Verification items for the finished model (mm, model axes). Face numbers are marked on the shaded views. A direction names the side the tool comes from. Give positions to 0.01 mm unless a question says otherwise; leave off trailing zeros. Write each loop counter-clockwise with the first axis right and the second up, starting at its lowest first coordinate (ties: lowest second). Pieces come first, ordered by that corner, then holes. Notation, with made-up numbers: (55.25, -3) -> (94.25, -3) arc R8 ccw to (94.25, 4) -> close; hole circle Ø1 at (46, 45). An arc over 180 degrees is marked (long way). Answer as CSV lines item,"result".
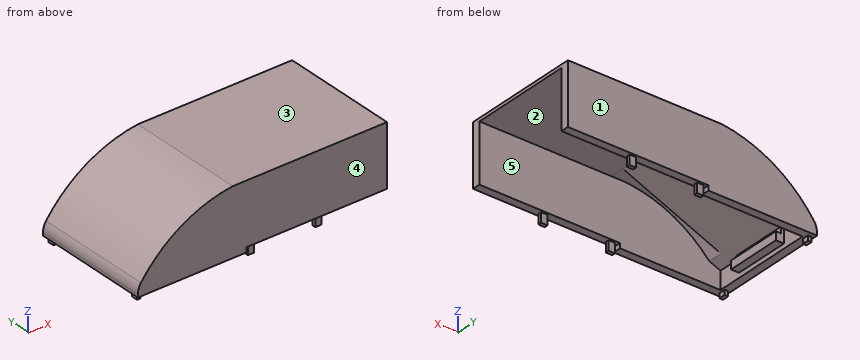
```python
from build123d import *

# Parameters (mm, degrees)
CROQUIS1_W              = 118
CROQUIS1_H              = 74
SALIENTE_EXTRUIR1_DEPTH = 36
CROQUIS2_W              = 36
CROQUIS2_H              = 64
CORTAR_EXTRUIR1_DEPTH   = 120
CORTAR_EXTRUIR3_DEPTH   = 102.257098517
SALIENTE_EXTRUIR2_DEPTH = 64
CORTAR_EXTRUIR4_DEPTH   = 9
CORTAR_EXTRUIR5_DEPTH   = 9
SALIENTE_EXTRUIR4_DEPTH = 5
CROQUIS14_W             = 50.5
CROQUIS14_H             = 3
CORTAR_EXTRUIR7_DEPTH   = 74
CROQUIS15_W             = 4
CROQUIS15_H             = 2.2
CROQUIS15_W_2           = 2.2
CROQUIS15_H_2           = 4
SALIENTE_EXTRUIR3_DEPTH = 6
REDONDEO1_R             = 10
SALIENTE_EXTRUIR5_DEPTH = 37
CROQUIS21_W             = 8
CROQUIS21_H             = 35
SALIENTE_EXTRUIR6_DEPTH = 5
CROQUIS22_W             = 2.9
CROQUIS22_H             = 35
CORTAR_EXTRUIR8_DEPTH   = 5
CROQUIS23_W             = 3.8
CROQUIS23_H             = 35
SALIENTE_EXTRUIR7_DEPTH = 1.9


with BuildPart() as part:
    # Croquis1 → Saliente-Extruir1 (new body)
    with BuildSketch(Plane.XY):
        Rectangle(CROQUIS1_W, CROQUIS1_H)
    extrude(amount=SALIENTE_EXTRUIR1_DEPTH)

    # Croquis2 → Cortar-Extruir1 (cut)
    with BuildSketch(Plane(origin=(59, 0, 0), x_dir=(0, 0, -1), z_dir=(1, 0, 0))):
        with Locations((-18, 0)):
            Rectangle(CROQUIS2_W, CROQUIS2_H)
    extrude(amount=-CORTAR_EXTRUIR1_DEPTH, mode=Mode.SUBTRACT)


with BuildPart() as cortar_extruir1_piece_1:
    # of the separate pieces the step leaves, piece 1, a body of its own (cortar_extruir1_pieces)
    add(part.part.solids().sort_by_distance((-59, 37, 0))[0])


with BuildPart() as cortar_extruir1_piece_2:
    # of the separate pieces the step leaves, piece 2, a body of its own (cortar_extruir1_pieces)
    add(part.part.solids().sort_by_distance((-59, -37, 0))[0])


with BuildPart() as cortar_extruir3_tool:
    # Croquis6 → Cortar-Extruir3 (new, through all)
    with BuildSketch(Plane.XZ.offset(37)):
        with BuildLine():
            Line((-59, 0), (-59, 36))
            Line((-59, 36), (0, 36))
            ThreePointArc((0, 36), (-33.535731191, 24.614115008), (-59, 0))
        make_face()
    extrude(amount=-CORTAR_EXTRUIR3_DEPTH)


with BuildPart() as cortar_extruir1_piece_1_1:
    add(cortar_extruir1_piece_1.part)

    # Cortar-Extruir3: cut by cortar_extruir3_tool
    add(cortar_extruir3_tool.part, mode=Mode.SUBTRACT)



with BuildPart() as cortar_extruir1_piece_2_1:
    add(cortar_extruir1_piece_2.part)

    # Cortar-Extruir3: cut by cortar_extruir3_tool
    add(cortar_extruir3_tool.part, mode=Mode.SUBTRACT)


with BuildPart() as cortar_extruir1_piece_1_2:
    add(cortar_extruir1_piece_1_1.part)

    add(cortar_extruir1_piece_2_1.part)  # Saliente-Extruir2 merges Cortar-Extruir1 piece 2
    # Croquis7 → Saliente-Extruir2 (add)
    with BuildSketch(Plane.XZ.offset(-32)):
        with BuildLine():
            Line((0, 36), (59, 36))
            Line((59, 36), (59, 34))
            Line((59, 34), (14, 34))
            Line((14, 34), (-54, 6))
            Line((-54, 6), (-54, 0))
            Line((-54, 0), (-59, 0))
            ThreePointArc((-59, 0), (-33.535731191, 24.614115008), (0, 36))
        make_face()
    extrude(amount=SALIENTE_EXTRUIR2_DEPTH)

    # Croquis8 → Cortar-Extruir4 (cut)
    with BuildSketch(Plane.XZ.offset(-32)):
        with BuildLine():
            Line((14, 34), (-46.937159353, 8.908228502))
            ThreePointArc((-46.937159353, 8.908228502), (-19.288572578, 28.30266844), (14, 34))
        make_face()
    extrude(amount=CORTAR_EXTRUIR4_DEPTH, mode=Mode.SUBTRACT)

    # Croquis13 → Cortar-Extruir5 (cut)
    with BuildSketch(Plane(origin=(0, -32, 0), x_dir=(1, 0, 0), z_dir=(0, 1, 0))):
        with BuildLine():
            Line((14, -34), (-46.936286689, -8.908587834))
            ThreePointArc((-46.936286689, -8.908587834), (-19.28805118, -28.302641518), (14, -34))
        make_face()
    extrude(amount=CORTAR_EXTRUIR5_DEPTH, mode=Mode.SUBTRACT)

    # Croquis17 → Saliente-Extruir4 (add)
    with BuildSketch(Plane(origin=(0, 0, 0), x_dir=(-1, 0, 0), z_dir=(0, 0, -1))):
        Polygon((-59, 37), (-59, 32), (54, 32), (54, -32), (-59, -32), (-59, -37), (59, -37), (59, 37), align=None)
    extrude(amount=SALIENTE_EXTRUIR4_DEPTH)

    # Croquis14 → Cortar-Extruir7 (cut)
    with BuildSketch(Plane.XZ.offset(37)):
        with Locations((33.75, -3.5)):
            Rectangle(CROQUIS14_W, CROQUIS14_H)
    extrude(amount=-CORTAR_EXTRUIR7_DEPTH, mode=Mode.SUBTRACT)

    # Croquis15 → Saliente-Extruir3 (add)
    with BuildSketch(Plane(origin=(0, 0, -2), x_dir=(-1, 0, 0), z_dir=(0, 0, -1))):
        with Locations((-54.5, 34.5)):
            Rectangle(CROQUIS15_W, CROQUIS15_H)
        with Locations((-54.5, -34.5)):
            Rectangle(CROQUIS15_W, CROQUIS15_H)
        with Locations((-12.5, 34.5)):
            Rectangle(CROQUIS15_W, CROQUIS15_H)
        with Locations((-12.5, -34.5)):
            Rectangle(CROQUIS15_W, CROQUIS15_H)
        with Locations((56.5, -32.5)):
            Rectangle(CROQUIS15_W_2, CROQUIS15_H_2)
        with Locations((56.5, 32.5)):
            Rectangle(CROQUIS15_W_2, CROQUIS15_H_2)
    extrude(amount=SALIENTE_EXTRUIR3_DEPTH)

    # Redondeo1
    redondeo1_edges = [cortar_extruir1_piece_1_2.edges().sort_by_distance(p)[0] for p in [
        (-59, 0, 0),
    ]]
    fillet(redondeo1_edges, radius=REDONDEO1_R)

    # Croquis19 → Saliente-Extruir5 (add)
    with BuildSketch(Plane(origin=(59, 0, 0), x_dir=(0, 0, -1), z_dir=(1, 0, 0))):
        Polygon((2, 37), (2, 32), (-34, 32), (-34, -32), (2, -32), (2, -37), (-36, -37), (-36, 37), align=None)
    extrude(amount=SALIENTE_EXTRUIR5_DEPTH)

    # Croquis21 → Saliente-Extruir6 (add)
    with BuildSketch(Plane(origin=(-54, 0, 0), x_dir=(0, 0, -1), z_dir=(1, 0, 0))):
        with Locations((1, 0.003682439)):
            Rectangle(CROQUIS21_W, CROQUIS21_H)
    extrude(amount=SALIENTE_EXTRUIR6_DEPTH)

    # Croquis22 → Cortar-Extruir8 (cut)
    with BuildSketch(Plane(origin=(-49, 0, 0), x_dir=(0, 0, -1), z_dir=(1, 0, 0))):
        with Locations((3.55, 0.003682439)):
            Rectangle(CROQUIS22_W, CROQUIS22_H)
    extrude(amount=-CORTAR_EXTRUIR8_DEPTH, mode=Mode.SUBTRACT)

    # Croquis23 → Saliente-Extruir7 (add)
    with BuildSketch(Plane(origin=(-54, 0, 0), x_dir=(0, 0, -1), z_dir=(1, 0, 0))):
        with Locations((-4.9, 0.003682439)):
            Rectangle(CROQUIS23_W, CROQUIS23_H)
    extrude(amount=SALIENTE_EXTRUIR7_DEPTH)


solid = cortar_extruir1_piece_1_2.part
```
1) Section check B-B (x = 70). Record the boundary of the cut face in (y, z).
Reported:
outline,"(-37, -2) -> (-32, -2) -> (-32, 34) -> (32, 34) -> (32, -2) -> (37, -2) -> (37, 36) -> (-37, 36) -> close"
2) Section check A-A (y = -7). Record the boundary of the cut face in (x, z).
Reported:
outline,"(-59, -5) -> (-54, -5) -> (-54, -2.1) -> (-49, -2.1) -> (-49, 3) -> (-52.1, 3) -> (-52.1, 6.78) -> (14, 34) -> (96, 34) -> (96, 36) -> (0, 36) arc R80.94 ccw to (-57.12, 2.73) arc R10 ccw to (-59, -3.1) -> close"
3) Scan lines: line 1 along Y through (x, z) = (-40, 12.5); line 2 along Y through (x, z) = (40, 31.5); line 3 along Z through (x, y) = (78, 20). Record each from-to range of solid material in increasing order.
Reported:
line 1,"-37 to -32, -23 to 23, 32 to 37"
line 2,"-37 to -32, 32 to 37"
line 3,"34 to 36"
4) Tool access check on the marked faces 1 and 2. Record the directions out of +Z, -Z, +X, -X, +Y, -Y that give a thin tool (end or side, any length) a straight path to the whole face; none if there is none.
Reported:
face 1,"+Z, -Z, +X, -X, +Y"
face 2,"-Z, +X"
5) Section check D-D (y = -19.5). Record the boundary of the cut face in (x, z), and give its area (3 significant figures).
Reported:
outline,"(-59, -5) -> (-54, -5) -> (-54, 6) -> (14, 34) -> (96, 34) -> (96, 36) -> (0, 36) arc R80.94 ccw to (-57.12, 2.73) arc R10 ccw to (-59, -3.1) -> close"
area,"755 mm²"
6) Depth check by flat-ended pin: pin 1 (2.5 mm diameter, centred on x = 40.5, y = 34.5, fed in from -Z); pin 2 (2.5 mm diameter, centred on y = 32.5, z = -7, fed in from -X); pin 3 (19 mm diameter, centred on x = 63, y = -12, fed in from -Z). Enter the tip coordinate at first touch or a pass-through.
Reported:
pin 1,"z = -2"
pin 2,"x = -57.6"
pin 3,"z = 34"
7) Section check C-C (z = 15). Record the boundary of the cut face in (x, y).
Reported:
outline,"(-46.27, -37) -> (96, -37) -> (96, -32) -> (-40.73, -32) -> (-40.73, -23) -> (-32.14, -23) -> (-32.14, 23) -> (-40.73, 23) -> (-40.73, 32) -> (96, 32) -> (96, 37) -> (-46.27, 37) -> close"
8) Draft check along Y on the marked faces 3, 4 and 5. Enter one of: +Y half, -Y half, draft (parallel to the pull), parting line (faces both ways), or undercut.
Reported:
face 3,"draft"
face 4,"-Y half"
face 5,"undercut"
